Model file for the job. Use its own axes, mm. Face numbers are marked on the shaded views. A direction names the side the tool comes from. Give positions to 0.01 mm unless a question says otherwise; leave off trailing zeros. Write each loop counter-clockwise with the first axis right and the second up, starting at its lowest first coordinate (ties: lowest second). Pieces come first, ordered by that corner, then holes. Notation, with made-up numbers: (-11, -31) - (25, -31) arc R14 cw to (25, -6) - close; hole circle Ø7 at (58.25, 47). An arc over 180 degrees is marked (long way). One line per item, written item: value. Start each with the question number.
(1) Cut at D-D, the plane y = 7. State how many separate pieces and enclosed holes the cut face has, and give its area (3 significant figures).
(2) Drop flat-ended pins along their axis: P1, Ø1.5, axis at x = -32, z = -18.5, coming from the -Y side; P2, Ø5, axis at y = -0.5, z = 14, coming from the +X side; P3, Ø10, axis at x = 17, z = 5.5, coming from the +Y side (3 decimals); P4, Ø6, axis at x = 15, y = 5.5, coming from the -Z side. Give the stop position or say it passes through.
(3) 3-axis set-ups, long thin cutter, end or side, ignore diameter. For the marked faces 5, 6, 7, 8 and 9: which of +Z, -Z, +X, -X, +Y, -Y reach the whole face in a straight line?
(4) Probe L1, parallel to X at y = -16.5, z = 0 (3 decimals); L2, parallel to Y at x = -0.5, z = 14.5 (3 decimals); L3, parallel to X at y = 7, z = 17. List the from-to ranges inside material, lowest first.
(5) Mould opens along Z. For the marked faces 1, 2, 3 and 4 say: pulls with the +Z half, pulls with the -Z half, needs draft (parallel to the pull), parting line crosses it, or undercut.
(6) Cut at C-C, the plane y = -27. List the corners of the cut face in (x, z) (3 decimals), and give its area (3 significant figures).
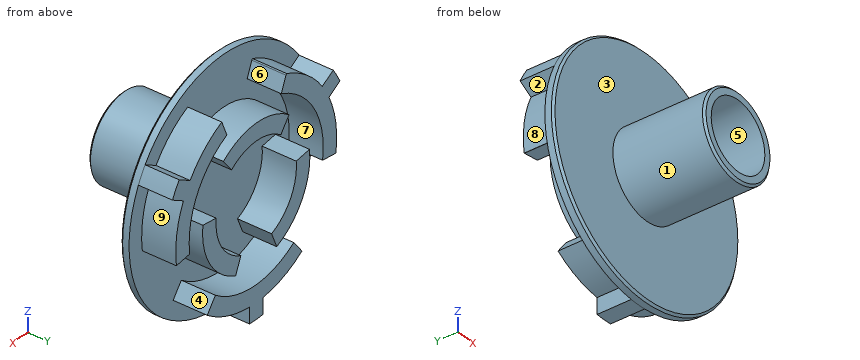
from build123d import *

# Parameters (mm, degrees)
SKETCH1_R           = 44.05249
BOSS_EXTRUDE1_DEPTH = 3.175
SKETCH2_R           = 15.875
BOSS_EXTRUDE2_DEPTH = 34.12998
SKETCH3_R           = 25.4
SKETCH3_R_2         = 19.05
BOSS_EXTRUDE3_DEPTH = 12.7
CUT_EXTRUDE2_DEPTH  = 73.614773175
CIRPATTERN1_COUNT   = 3
SKETCH5_R           = 38.1
SKETCH5_R_2         = 31.75
BOSS_EXTRUDE5_DEPTH = 12.7
CUT_EXTRUDE4_DEPTH  = 12.7
CIRPATTERN3_COUNT   = 3
BOSS_EXTRUDE6_DEPTH = 12.7
CIRPATTERN4_COUNT   = 3
SKETCH8_R           = 12.7
CUT_EXTRUDE5_DEPTH  = 34.12998
CHAMFER1_SIZE       = 0.762


with BuildPart() as part:
    # Sketch1 → Boss-Extrude1 (new body)
    with BuildSketch(Plane(origin=(0, 0, 0), x_dir=(1, 0, 0), z_dir=(0, 1, 0))):
        with Locations(Location((0, 0, 0), (0, 0, 270))):
            Circle(SKETCH1_R)
    extrude(amount=BOSS_EXTRUDE1_DEPTH)

    # Sketch2 → Boss-Extrude2 (add)
    with BuildSketch(Plane.XZ):
        with Locations(Location((0, 0, 0), (0, 0, 270))):
            Circle(SKETCH2_R)
    extrude(amount=BOSS_EXTRUDE2_DEPTH)

    # Sketch3 → Boss-Extrude3 (add)
    with BuildSketch(Plane(origin=(0, 3.175, 0), x_dir=(1, 0, 0), z_dir=(0, 1, 0))):
        with Locations(Location((0, 0, 0), (0, 0, 270))):
            Circle(SKETCH3_R)
        with Locations(Location((0, 0, 0), (0, 0, 270))):
            Circle(SKETCH3_R_2, mode=Mode.SUBTRACT)
    extrude(amount=BOSS_EXTRUDE3_DEPTH)

    # Sketch4 → Cut-Extrude2 (cut, through all)
    with BuildSketch(Plane(origin=(0, 3.175, 0), x_dir=(1, 0, 0), z_dir=(0, 1, 0))):
        Polygon((0, 0), (11.462134213, 27.672039871), (-12.066850466, 29.13195405), align=None)
    cut_extrude2 = extrude(amount=CUT_EXTRUDE2_DEPTH, mode=Mode.SUBTRACT)

    # CirPattern1: Cut-Extrude2 ×3 about axis
    cirpattern1_axis = Axis((0, 0, -0.454253878), (0, 1, 0))
    for i in range(1, CIRPATTERN1_COUNT):
        add(cut_extrude2.rotate(cirpattern1_axis, i * 360 / CIRPATTERN1_COUNT), mode=Mode.SUBTRACT)

    # Sketch5 → Boss-Extrude5 (add)
    with BuildSketch(Plane(origin=(0, 3.175, 0), x_dir=(1, 0, 0), z_dir=(0, 1, 0))):
        with Locations(Location((0, 0, 0), (0, 0, 270))):
            Circle(SKETCH5_R)
        with Locations(Location((0, 0, 0), (0, 0, 270))):
            Circle(SKETCH5_R_2, mode=Mode.SUBTRACT)
    extrude(amount=BOSS_EXTRUDE5_DEPTH)

    # Sketch6 → Cut-Extrude4 (cut)
    with BuildSketch(Plane(origin=(0, 15.875, 0), x_dir=(1, 0, 0), z_dir=(0, 1, 0))):
        Polygon((24.518856113, 31.953595399), (30.847960217, 40.201844455), (52.890000535, 5.212460302), (39.592566776, 5.212460302), (30.847960217, 4.061211008), (18.173239697, 23.68382708), align=None)
    cut_extrude4 = extrude(amount=-CUT_EXTRUDE4_DEPTH, mode=Mode.SUBTRACT)

    # CirPattern3: Cut-Extrude4 ×3 about axis
    cirpattern3_axis = Axis((1.188980204, 0, -0.687015275), (0, 1, 0))
    for i in range(1, CIRPATTERN3_COUNT):
        add(cut_extrude4.rotate(cirpattern3_axis, i * 360 / CIRPATTERN3_COUNT), mode=Mode.SUBTRACT)

    # Sketch7 → Boss-Extrude6 (add)
    with BuildSketch(Plane(origin=(0, 3.175, 0), x_dir=(1, 0, 0), z_dir=(0, 1, 0))):
        with BuildLine():
            Line((3.175, 35.86061982), (3.175, 43.937924965))
            ThreePointArc((3.175, 43.937924965), (0, 44.05249), (-3.175, 43.937924965))
            Line((-3.175, 43.937924965), (-3.175, 35.86061982))
            ThreePointArc((-3.175, 35.86061982), (0, 36.000898307), (3.175, 35.86061982))
        make_face()
    boss_extrude6 = extrude(amount=BOSS_EXTRUDE6_DEPTH)

    # CirPattern4: Boss-Extrude6 ×3 about axis
    cirpattern4_axis = Axis((0, 0, 0), (0, 1, 0))
    for i in range(1, CIRPATTERN4_COUNT):
        add(boss_extrude6.rotate(cirpattern4_axis, i * 360 / CIRPATTERN4_COUNT))

    # Sketch8 → Cut-Extrude5 (cut)
    with BuildSketch(Plane.XZ.offset(34.12998)):
        with Locations(Location((0, 0, 0), (0, 0, 270))):
            Circle(SKETCH8_R)
    extrude(amount=-CUT_EXTRUDE5_DEPTH, mode=Mode.SUBTRACT)

    # Chamfer1
    chamfer1_edges = [part.edges().sort_by_distance(p)[0] for p in [
        (0, 0, -44.05249),
        (0, -34.12998, 15.875),
    ]]
    chamfer(chamfer1_edges, length=CHAMFER1_SIZE)


solid = part.part
Answers follow:
1. separate pieces: 6
1. enclosed holes: 0
1. area: 1,510 mm²
2. P1: stops at y = 0
2. P2: stops at x = 42.43
2. P3: stops at y = 15.875
2. P4: stops at z = -42.06
3. face 5: -Y
3. face 6: +Z, +Y
3. face 7: +Y
3. face 8: -X, +Y
3. face 9: +X, +Y
4. L1: x = -15.875 to -12.7, 12.7 to 15.875
4. L2: y = -34.13 to 3.175
4. L3: x = -35.79 to -26.82, -13.17 to -8.6, 8.6 to 13.17, 26.82 to 35.79
5. face 1: parting line crosses it
5. face 2: undercut
5. face 3: needs draft
5. face 4: undercut
6. outline: circle Ø31.75 at (0, 0); hole circle Ø25.4 at (0, 0)
6. area: 285 mm²
